from build123d import *

# Parameters (mm, degrees)
BOSS_EXTRUDE1_DEPTH      = 1
BOSS_EXTRUDE1_DEPTH_BACK = 3
SKETCH3_R                = 14
SKETCH6_R                = 3.05
CUT_EXTRUDE2_DEPTH       = 1.1
BOSS_EXTRUDE2_DEPTH      = 2
CUT_EXTRUDE3_DEPTH       = 3


with BuildPart() as part:
    # Sketch3 → Boss-Extrude1 (new, two sides: drawn at the far end of the back side and taken through both)
    with BuildSketch(Plane.XY.offset(-51.612811659).offset(-BOSS_EXTRUDE1_DEPTH_BACK)):
        with Locations((0, 8)):
            Circle(SKETCH3_R)
    extrude(amount=BOSS_EXTRUDE1_DEPTH + BOSS_EXTRUDE1_DEPTH_BACK)

    # Sketch6 → Cut-Extrude2 (cut)
    with BuildSketch(Plane.XY.offset(-50.612811659)):
        Circle(SKETCH6_R)
        with Locations(Location((0, 16, 0), (0, 0, 180))):
            Circle(SKETCH6_R)
    extrude(amount=-CUT_EXTRUDE2_DEPTH, mode=Mode.SUBTRACT)

    # Sketch7 → Boss-Extrude2 (add)
    with BuildSketch(Plane.XY.offset(-50.612811659)):
        with BuildLine():
            Line((-8, 9), (-8, 7))
            ThreePointArc((-8, 7), (-9, 6), (-10, 7))
            Line((-10, 7), (-10, 9))
            ThreePointArc((-10, 9), (-9, 10), (-8, 9))
        make_face()
        with BuildLine():
            Line((8, 9), (8, 7))
            ThreePointArc((8, 7), (9, 6), (10, 7))
            Line((10, 7), (10, 9))
            ThreePointArc((10, 9), (9, 10), (8, 9))
        make_face()
    extrude(amount=BOSS_EXTRUDE2_DEPTH)

    # Sketch8 → Cut-Extrude3 (cut)
    with BuildSketch(Plane(origin=(0, 0, -54.612811659), x_dir=(-1, 0, 0), z_dir=(0, 0, -1))):
        with BuildLine():
            Line((-1.55, 10.024845673), (-1.55, 5.975154327))
            ThreePointArc((-1.55, 5.975154327), (0, 5.45), (1.55, 5.975154327))
            Line((1.55, 5.975154327), (1.55, 10.024845673))
            ThreePointArc((1.55, 10.024845673), (0, 10.55), (-1.55, 10.024845673))
        make_face()
    extrude(amount=-CUT_EXTRUDE3_DEPTH, mode=Mode.SUBTRACT)


solid = part.part
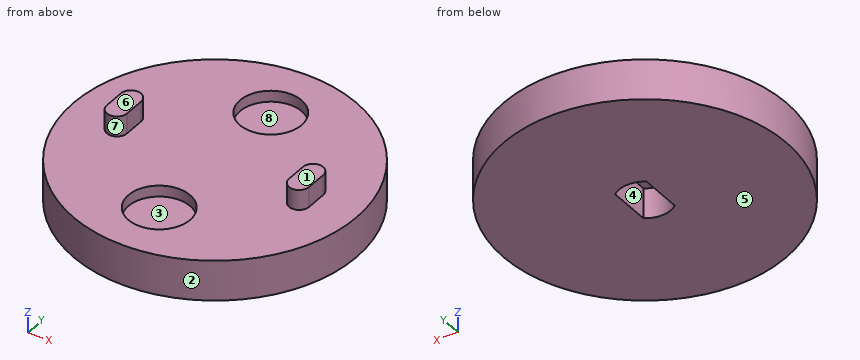
Verification items for the finished model (mm, model axes). Face numbers are marked on the shaded views. A direction names the side the tool comes from. Round coordinates to 2 decimals unless told otherwise and drop trailing zeros. Write each loop counter-clockwise with the first axis right and the second up, starting at its lowest first coordinate (ties: lowest second). Pieces come first, ordered by that corner, then holes.
(1) Section check C-C (x = 0). Enter the section's corners in (y, z).
Returned:
outline: (-6, -54.61) - (5.45, -54.61) - (5.45, -51.61) - (10.55, -51.61) - (10.55, -54.61) - (22, -54.61) - (22, -50.61) - (19.05, -50.61) - (19.05, -51.71) - (12.95, -51.71) - (12.95, -50.61) - (3.05, -50.61) - (3.05, -51.71) - (-3.05, -51.71) - (-3.05, -50.61) - (-6, -50.61) - close
(2) Section check B-B (y = 8). Enter the section's corners in (x, z).
Returned:
outline: (-14, -54.61) - (-1.55, -54.61) - (-1.55, -51.61) - (1.55, -51.61) - (1.55, -54.61) - (14, -54.61) - (14, -50.61) - (10, -50.61) - (10, -48.61) - (8, -48.61) - (8, -50.61) - (-8, -50.61) - (-8, -48.61) - (-10, -48.61) - (-10, -50.61) - (-14, -50.61) - close
(3) Depth check by flat-ended pin: pin 1 Ø1 at (y, z) = (8, -49.5) entering from -X; pin 2 Ø0.6 at (y, z) = (8.5, -50) entering from +X; pin 3 Ø6.5 at (x, y) = (0, 16.5) entering from +Z. Enter the tip coordinate at first touch or a pass-through.
Returned:
pin 1: stops at x = -10
pin 2: stops at x = 10
pin 3: stops at z = -50.61
(4) Access from +Z, -Z, +X, -X, +Y, -Y to the whole of each face (thin tool, end or side, straight path). Record for the marked faces 4, 5, 6, 7 and 8.
Returned:
face 4: -Z
face 5: -Z, +X, -X, +Y, -Y
face 6: +Z, +X, -X, +Y, -Y
face 7: +Z, -Y
face 8: +Z
(5) Mould release check, pull along X, two halves, no side actions. Record for the marked faces 1, 2 and 3: pulls with the +X half, pulls with the -X half, needs draft (parallel to the pull), parting line crosses it, or undercut.
Returned:
face 1: needs draft
face 2: parting line crosses it
face 3: undercut
(6) Section check A-A (z = -48.95). Enter the section's corners in (x, y), plus the area to 3 significant figures.
Returned:
outline: (-10, 7) arc R1 ccw to (-8, 7) - (-8, 9) arc R1 ccw to (-10, 9) - close; (8, 7) arc R1 ccw to (10, 7) - (10, 9) arc R1 ccw to (8, 9) - close
area: 14.3 mm2
(7) Material ranges on line 1 (Y direction, x = 0, z = -50.9); line 2 (Z direction, x = 0.25, y = 13); line 3 (Z direction, x = -6, y = 16.5), recorded low to high.
Returned:
line 1: y = -6 to -3.05, 3.05 to 12.95, 19.05 to 22
line 2: z = -54.61 to -51.71
line 3: z = -54.61 to -50.61
(8) Section check D-D (x = 8.5). Enter the section's corners in (y, z).
Returned:
outline: (-3.12, -54.61) - (19.12, -54.61) - (19.12, -50.61) - (9.87, -50.61) - (9.87, -48.61) - (6.13, -48.61) - (6.13, -50.61) - (-3.12, -50.61) - close
